Model file for the job. Use its own axes, mm. A direction names the side the tool comes from. Round coordinates to 2 decimals unless told otherwise and drop trailing zeros. Loops run counter-clockwise (first coordinate to the right, second up) from the corner with the lowest first, then second, coordinate; pieces in that order, holes last.
from build123d import *

# Parameters (mm, degrees)
SKETCH_1_R               = 12
EXTRUDE_1_DEPTH          = 2.5
SKETCH_2_R               = 5.7
CUT_EXTRUDE_1_DEPTH      = 2.5
SKETCH_3_R               = 7
EXTRUDE_2_DEPTH          = 6
CUT_EXTRUDE_3_DEPTH      = 19.980252896
CUT_EXTRUDE_START        = -3
SKETCH_6_R               = 5.7
CUT_EXTRUDE_4_DEPTH      = 3
SKETCH_12_R              = 1.5
CUT_EXTRUDE_7_DEPTH      = 8.5
PATTERN_CIRCULAR_3_COUNT = 3
SKETCH_16_W              = 4.841129394
SKETCH_16_H              = 2.5
EXTRUDE_5_DEPTH          = 5
PATTERN_CIRCULAR_4_COUNT = 3


with BuildPart() as part:
    # Sketch 1 → Extrude 1 (new body)
    with BuildSketch(Plane(origin=(0, 0, 0), x_dir=(1, 0, 0), z_dir=(0, 1, 0))):
        with Locations(Location((0, 0, 0), (0, 0, 270))):
            Circle(SKETCH_1_R)
    extrude(amount=EXTRUDE_1_DEPTH)

    # Sketch 2 → Cut-Extrude 1 (cut)
    with BuildSketch(Plane(origin=(0, 2.5, 0), x_dir=(1, 0, 0), z_dir=(0, 1, 0))):
        with Locations(Location((0, 0, 0), (0, 0, 270))):
            Circle(SKETCH_2_R)
    extrude(amount=-CUT_EXTRUDE_1_DEPTH, mode=Mode.SUBTRACT)

    # Sketch 3 → Extrude 2 (add)
    with BuildSketch(Plane(origin=(0, 2.5, 0), x_dir=(1, 0, 0), z_dir=(0, 1, 0))):
        with Locations(Location((0, 0, 0), (0, 0, 270))):
            Circle(SKETCH_3_R)
    extrude(amount=EXTRUDE_2_DEPTH)

    # Sketch 5 → Cut-Extrude 3 (cut, through all)
    with BuildSketch(Plane(origin=(0, 8.5, 0), x_dir=(1, 0, 0), z_dir=(0, 1, 0))):
        Polygon((3.334197805, -1.925), (3.334197805, 1.925), (0, 3.85), (-3.334197805, 1.925), (-3.334197805, -1.925), (0, -3.85), align=None)
    extrude(amount=-CUT_EXTRUDE_3_DEPTH, mode=Mode.SUBTRACT)

    # Sketch 6 → Cut-Extrude 4 (cut)
    with BuildSketch(Plane.XZ.offset(-2.5).offset(CUT_EXTRUDE_START)):
        with Locations(Location((0, 0, 0), (0, 0, 90))):
            Circle(SKETCH_6_R)
    extrude(amount=CUT_EXTRUDE_4_DEPTH, mode=Mode.SUBTRACT)

    # Sketch 12 → Cut-Extrude 7 (cut)
    with BuildSketch(Plane(origin=(0, 0, 0), x_dir=(-1, 0, 0), z_dir=(0, -1, 0))):
        with Locations(Location((-4.46, 7.724946602, 0), (0, 0, 90))):
            Circle(SKETCH_12_R)
    cut_extrude_7 = extrude(amount=-CUT_EXTRUDE_7_DEPTH, mode=Mode.SUBTRACT)

    # Pattern Circular 3: Cut-Extrude 7 ×3 about axis
    pattern_circular_3_axis = Axis((0, 0, 0), (0, 1, 0))
    for i in range(1, PATTERN_CIRCULAR_3_COUNT):
        add(cut_extrude_7.rotate(pattern_circular_3_axis, i * 360 / PATTERN_CIRCULAR_3_COUNT), mode=Mode.SUBTRACT)

    # Sketch 16 → Extrude 5 (add)
    with BuildSketch(Plane(origin=(0, 2.5, 0), x_dir=(1, 0, 0), z_dir=(0, 1, 0))):
        with Locations((8.734133088, -0.110223506)):
            Rectangle(SKETCH_16_W, SKETCH_16_H)
    extrude_5 = extrude(amount=EXTRUDE_5_DEPTH)

    # Pattern Circular 4: Extrude 5 ×3 about axis
    pattern_circular_4_axis = Axis((0, 0, 0), (0, 1, 0))
    for i in range(1, PATTERN_CIRCULAR_4_COUNT):
        add(extrude_5.rotate(pattern_circular_4_axis, i * 360 / PATTERN_CIRCULAR_4_COUNT))


solid = part.part
Q1. Slice it at C-C on x = 4.46. Give the cut face in (y, z).
Q2. Flat gauge pins, fed straight in: P1, Ø10.5, axis at x = 0, z = 0, coming from the -Y side; P2, Ø1.5, axis at x = -1.5, y = 1.5, coming from the +Z side; P3, Ø2.5, axis at y = 6.5, z = 0.5, coming from the -X side. Where does each tip first touch, or does it go through?
Q3. Tool access for faces 1 (the face through (-3.5, 2.8, -4.5)), 2 (the face through (9, 5, 1.36)), 3 (the face through (-1.69, 7.021, 2.874)), 4 (the face through (-4, 7.5, -8)): list every direction of +Z, -Z, +X, -X, +Y, -Y with a clear straight run to the whole face (end or side of a thin tool).
Q4. Slice it at B-B on z = 0. Give the cut face in (x, y).
Q5. Probe line 1 (Z direction, x = -6, y = 7); line 2 (X direction, y = 1.75, z = -0.25); line 3 (Z direction, x = -5.25, y = 5.75). List the from-to ranges inside material, lowest first.
Q6. Pull direction Y, two halves, no side cores. Call faces 5 (the face through (-5.688, 4.965, 9.596)), 6 (the face through (2, 5.5, -3)), 7 (the face through (-5, 7.5, 8)): pulls with the +Y half, pulls with the -Y half, needs draft (parallel to the pull), parting line crosses it, or undercut.
Q7. Slice it at D-D on x = -8.92. Give the cut face in (y, z), plus the area to 3 significant figures.
Q8. Slice it at A-A on y = 3.25. Give the cut face in (x, z), plus the area to 3 significant figures.
Reply:
1. outline: (0, -11.14) - (2.5, -11.14) - (2.5, -9.22) - (0, -9.22) - close; (0, -6.22) - (2.5, -6.22) - (2.5, -5.4) - (8.5, -5.4) - (8.5, 5.4) - (2.5, 5.4) - (2.5, 6.22) - (0, 6.22) - (0, 3.55) - (5.5, 3.55) - (5.5, -3.55) - (0, -3.55) - close; (0, 9.22) - (2.5, 9.22) - (2.5, 11.14) - (0, 11.14) - close
2. P1: stops at y = 5.5
2. P2: stops at z = 11.98
2. P3: stops at x = -7
3. face 1: -Y
3. face 2: +Z, +X, +Y
3. face 3: +Y, -Y
3. face 4: -Z, -X, +Y
4. outline: (-12, 0) - (-10.42, 0) - (-10.42, 2.5) - (-12, 2.5) - close; (-7.42, 0) - (-5.7, 0) - (-5.7, 5.5) - (-3.33, 5.5) - (-3.33, 8.5) - (-7, 8.5) - (-7, 2.5) - (-7.42, 2.5) - close; (3.33, 5.5) - (5.7, 5.5) - (5.7, 0) - (12, 0) - (12, 2.5) - (11.15, 2.5) - (11.15, 7.5) - (7, 7.5) - (7, 8.5) - (3.33, 8.5) - close
5. line 1: z = -9.42 to -8.11, -3.61 to 3.61, 7.67 to 9.42
5. line 2: x = -12 to -10.4, -7.44 to -5.69, 5.69 to 12
5. line 3: z = -9.85 to -6.81, -4.63 to 4.63, 6.37 to 9.85
6. face 5: needs draft
6. face 6: pulls with the -Y half
6. face 7: pulls with the +Y half
7. outline: (0, -8.03) - (2.5, -8.03) - (2.5, -1.5) - (0, -1.5) - close; (0, 1.5) - (2.5, 1.5) - (2.5, 8.03) - (0, 8.03) - close
7. area: 32.6 mm2
8. outline: (-6.76, 8.98) - (-4.61, 5.27) arc R7 ccw to (-4.44, -5.41) - (-6.56, -9.09) - (-4.4, -10.34) - (-2.26, -6.63) arc R7 ccw to (6.91, -1.14) - (11.15, -1.14) - (11.15, 1.36) - (6.87, 1.36) arc R7 ccw to (-2.47, 6.55) - (-4.59, 10.23) - close; hole circle Ø11.4 at (0, 0)
8. area: 83.3 mm2
